Input: part model. Units: mm. Frame: model coordinates. A direction names the side the tool comes from. Coordinates: 2 decimals unless noted, no trailing zeros. Loops run counter-clockwise (first coordinate to the right, second up) from the corner with the lowest first, then second, coordinate; pieces in that order, holes last.
Autodesk Inventor part; units mm, degrees
ref_plane "YZ Plane" through (0, 0, 0) normal (1, 0, 0) x (0, 1, 0)
ref_plane "XZ Plane" through (0, 0, 0) normal (0, 1, 0) x (-1, 0, 0)
ref_plane "XY Plane" through (0, 0, 0) normal (0, 0, 1) x (1, 0, 0)
sketch "スケッチ12" plane through (0, 0, 0) normal (0, 0, 1) x (1, 0, 0)
  circle A0 centre (0, 0) radius 30
  circle A1 centre (0, 0) radius 15
  line L0 (-30, 0) -> (30, 0)
  line L1 (-30, 0) -> (-11.8015, 50)
  line L2 (-11.8015, 50) -> (11.8015, 50)
  line L3 (11.8015, 50) -> (30, 0)
  circle A2 centre (0, 40) radius 3
  line L4 (11.8015, 50) -> (-30, 0)
  line L5 (-11.8015, 50) -> (30, 0)
  point P0 (22.9813, 19.2836)
  point P1 (-22.9813, 19.2836)
  point P2 (0, 51.9615)
  point P3 (5.316, 29.5252)
  point P4 (-5.316, 29.5252)
  point P5 (-2.2669, 48.0351)
  point P6 (2.2669, 48.0351)
  point P7 (0, 35.8839)
  point P8 (-15, 0)
  point P9 (15, 0)
  dimension "d5" = 60
  dimension "d6" = 30
  dimension "d10" = 70
  dimension "d11" = 70
  dimension "d12" = 50
  dimension "d13" = 40
  dimension "d14" = 6
  dimension "d38" = 30
extrude "押し出し2" add sketch "スケッチ12" along normal blind 10 contours L0 A1 A0 | L4 A0 L5 L0 A1 | A0 L1 | L1 A0 L4 | L3 A0 | L5 A0 L3 | L1 L5 A2 L4 A0 | L4 L5 A0 | A0 L5 L4 A2 L3 | L2 L4 A2 L5 | L5 A2 L4 picked at (0.1887, 36.6459)
sketch "スケッチ13" plane through (0, 0, 10) normal (0, 0, 1) x (1, 0, 0)
  circle A0 centre (0, 0) radius 20
  circle A1 centre (0, 0) radius 25
  circle A2 centre (0, 0) radius 22.5
  line L0 (0, 0) -> (-18.638, 32.282)
  line L1 (-18.638, 32.282) -> (0, 0)
  line L2 (0, 0) -> (-17.2844, -29.9374)
  line L3 (0, 0) -> (-56.8729, 0)
  line L4 (0, 0) -> (-31.7394, -18.3248)
  line L5 (0, 0) -> (-33.3883, 19.2767)
  line L6 (0, 0) -> (0, -31.9785)
  line L7 (0, 0) -> (-25.7143, 25.7143)
  line L8 (0, 0) -> (-33.0547, 8.857)
  line L9 (0, 0) -> (-32.621, -8.7408)
  line L10 (0, 0) -> (-23.652, -23.652)
  point P0 (-19.4856, 11.25)
  point P1 (-22.5, 0)
  point P2 (-19.4856, -11.25)
  point P3 (-11.25, -19.4856)
  point P4 (0, -22.5)
  point P5 (-16.5273, 4.4285)
  point P6 (-15.9099, 15.9099)
  point P7 (-21.7333, 5.8234)
  point P8 (-21.7333, -5.8234)
  point P9 (-15.9099, -15.9099)
  dimension "d19" = 45
  dimension "d17" = 40
  dimension "d18" = 50
  dimension "d20" = 60
  dimension "d21" = 60
  dimension "d22" = 30
  dimension "d23" = 30
  dimension "d31" = 150
  dimension "d32" = 15
  dimension "d34" = 15
  dimension "d35" = 15
  dimension "d36" = 15
hole "穴1" at (-15.9099, 15.9099, 10) at (-21.7333, 5.8234, 10) at (-21.7333, -5.8234, 10) at (-15.9099, -15.9099, 10) direction (0, 0, -1) diameter 3 end through all
sketch "スケッチ14" plane through (0, 0, 10) normal (0, 0, 1) x (1, 0, 0)
  circle A0 centre (-15.9099, 15.9099) radius 1.5
  circle A1 centre (-15.9099, 15.9099) radius 3
  circle A2 centre (-21.7333, 5.8234) radius 1.5
  circle A3 centre (-21.7333, 5.8234) radius 3
  circle A4 centre (-21.7333, -5.8234) radius 1.5
  circle A5 centre (-21.7333, -5.8234) radius 3
  circle A6 centre (-15.9099, -15.9099) radius 1.5
  circle A7 centre (-15.9099, -15.9099) radius 3
  point P0 (0, 0)
  dimension "d40" = 6
  dimension "d41" = 6
  dimension "d42" = 6
  dimension "d43" = 6
extrude "押し出し3" cut sketch "スケッチ14" against normal blind 4 contours A0 | A1 | A2 | A3 | A4 | A5 | A6 | A7
fillet "フィレット2" radius 15 2 edges at (-11.8015, 50, 5) (11.8015, 50, 5)
equation "\"d10\" = d11"
equation "\"d35\" = d34"
equation "\"d36\" = d35"
equation "\"d41\" = d40"
equation "\"d42\" = d41"
equation "\"d43\" = d42"
properties part number "legparts_04(six)"
Item 1: Contact query for flat-ended pins moving along their axis: P1, Ø3, axis at x = -22.5, y = -7, coming from the +Z side; P2, Ø1.5, axis at y = 28, z = 5, coming from the -X side; P3, Ø5, axis at y = -18, z = 7.5, coming from the -X side. Output: stop coordinate, or through.
Result:
P1: stops at z = 6
P2: stops at x = -20.08
P3: stops at x = -25.69
Item 2: Mould query, pull axis X, two halves, no side actions, for faces 3 (the face through (0, 50, 5)), 4 (the face through (-19.24, 29.56, 4.93)), 5 (the face through (-15.335, 14.524, 2.958)). Classes: +X half, -X half, draft (parallel to the pull), parting line (faces both ways), or undercut.
Result:
face 3: draft
face 4: -X half
face 5: undercut
Item 3: Section query D-D (x = 13.5). Output: boundary loops of the cut face in (y, z), then the cut area to 3 significant figures.
Result:
outline: (-26.79, 0) - (-6.54, 0) - (-6.54, 10) - (-26.79, 10) - close; (6.54, 0) - (43.72, 0) - (43.72, 10) - (6.54, 10) - close
area: 574 mm2
Item 4: Line query: L1, parallel to Y at x = 0, z = 2.75; L2, parallel to Y at x = 5, z = 2; L3, parallel to Y at x = -7.5, z = 6.5. Output: solid intervals per line, ascending.
Result:
L1: y = -30 to -15, 15 to 37, 43 to 50
L2: y = -29.58 to -14.14, 14.14 to 49.54
L3: y = -29.05 to -12.99, 12.99 to 48.66
Item 5: Reachability of faces 1 (the face through (0.953, -29.985, 4.93)), 2 (the face through (-14.6, -17.2, 6)) from +Z, -Z, +X, -X, +Y, -Y: full face, straight path, thin tool, end or side. Return the list, or none.
Result:
face 1: +Z, -Z
face 2: +Z
Item 6: Section query A-A (x = 0). Output: boundary loops of the cut face in (y, z).
Result:
outline: (-30, 0) - (-15, 0) - (-15, 10) - (-30, 10) - close; (15, 0) - (37, 0) - (37, 10) - (15, 10) - close; (43, 0) - (50, 0) - (50, 10) - (43, 10) - close
Item 7: Section query B-B (y = 0). Output: boundary loops of the cut face in (x, z).
Result:
outline: (-30, 0) - (-15, 0) - (-15, 10) - (-30, 10) - close; (15, 0) - (30, 0) - (30, 10) - (15, 10) - close
Item 8: Section query C-C (z = 2). Output: boundary loops of the cut face in (x, y).
Result:
outline: (-22.98, 19.28) arc R30 ccw (long way) to (22.98, 19.28) - (15.39, 40.13) arc R15 ccw to (1.3, 50) - (-1.3, 50) arc R15 ccw to (-15.39, 40.13) - close; hole circle Ø3 at (-21.73, -5.82); hole circle Ø3 at (-21.73, 5.82); hole circle Ø3 at (-15.91, -15.91); hole circle Ø3 at (-15.91, 15.91); hole circle Ø30 at (0, 0); hole circle Ø6 at (0, 40)
